```python
from build123d import *

# Parameters (mm, degrees)
BOSS_EXTRUDE1_START = 0.1
SKETCH1_R           = 3.884465816
BOSS_EXTRUDE1_DEPTH = 2.9
SKETCH2_R           = 3.884465816
SKETCH2_R_2         = 1.6
BOSS_EXTRUDE2_DEPTH = 1
SKETCH3_R           = 2.45
SKETCH3_R_2         = 1.6
BOSS_EXTRUDE3_DEPTH = 15.8


with BuildPart() as part:
    # Sketch1 → Boss-Extrude1 (new body)
    with BuildSketch(Plane.XY.offset(BOSS_EXTRUDE1_START)):
        with Locations((-0.001459351, 10.192904416)):
            Circle(SKETCH1_R)
        with BuildLine():
            Line((0.96845111, 13.081919272), (0.60411229, 12.721398629))
            ThreePointArc((0.60411229, 12.721398629), (0.587991908, 12.72520519), (0.571847603, 12.728908977))
            Line((0.571847603, 12.728908977), (0.404173908, 13.213267772))
            Line((0.404173908, 13.213267772), (0.114648145, 12.790310631))
            ThreePointArc((0.114648145, 12.790310631), (0.098098683, 12.790997601), (0.08154518, 12.791579126))
            Line((0.08154518, 12.791579126), (-0.174763937, 13.23545247))
            Line((-0.174763937, 13.23545247), (-0.379012427, 12.765345605))
            ThreePointArc((-0.379012427, 12.765345605), (-0.395392828, 12.762888154), (-0.411757242, 12.760326399))
            Line((-0.411757242, 12.760326399), (-0.747438103, 13.147671554))
            Line((-0.747438103, 13.147671554), (-0.859027247, 12.647405852))
            ThreePointArc((-0.859027247, 12.647405852), (-0.874646558, 12.641892799), (-0.89023043, 12.636280352))
            Line((-0.89023043, 12.636280352), (-1.293150653, 12.953097656))
            Line((-1.293150653, 12.953097656), (-1.308047329, 12.440754022))
            ThreePointArc((-1.308047329, 12.440754022), (-1.322341026, 12.432384623), (-1.336581115, 12.423924333))
            Line((-1.336581115, 12.423924333), (-1.792178114, 12.658763182))
            Line((-1.792178114, 12.658763182), (-1.709843917, 12.152859051))
            ThreePointArc((-1.709843917, 12.152859051), (-1.72229539, 12.141935797), (-1.734677021, 12.130933442))
            Line((-1.734677021, 12.130933442), (-2.226484333, 12.275306147))
            Line((-2.226484333, 12.275306147), (-2.049895036, 11.794126212))
            ThreePointArc((-2.049895036, 11.794126212), (-2.060054255, 11.781043899), (-2.070129925, 11.767897132))
            Line((-2.070129925, 11.767897132), (-2.580372352, 11.816585689))
            Line((-2.580372352, 11.816585689), (-2.315910352, 11.377521046))
            ThreePointArc((-2.315910352, 11.377521046), (-2.323410137, 11.362752503), (-2.330815684, 11.347936481))
            Line((-2.330815684, 11.347936481), (-2.841051735, 11.299181158))
            Line((-2.841051735, 11.299181158), (-2.498275379, 10.918100748))
            ThreePointArc((-2.498275379, 10.918100748), (-2.502844667, 10.902179748), (-2.507312436, 10.886229962))
            Line((-2.507312436, 10.886229962), (-2.999100852, 10.741792904))
            Line((-2.999100852, 10.741792904), (-2.590398969, 10.432469965))
            ThreePointArc((-2.590398969, 10.432469965), (-2.591872615, 10.415971935), (-2.593241129, 10.399464852))
            Line((-2.593241129, 10.399464852), (-3.048807394, 10.16456639))
            Line((-3.048807394, 10.16456639), (-2.588951536, 9.938180659))
            ThreePointArc((-2.588951536, 9.938180659), (-2.587276279, 9.921701881), (-2.585496075, 9.905234109))
            Line((-2.585496075, 9.905234109), (-2.988374839, 9.588364086))
            Line((-2.988374839, 9.588364086), (-2.493985393, 9.453097734))
            ThreePointArc((-2.493985393, 9.453097734), (-2.489221781, 9.437233793), (-2.484357202, 9.421400521))
            Line((-2.484357202, 9.421400521), (-2.819987375, 9.034011444))
            Line((-2.819987375, 9.034011444), (-2.308932865, 8.994753349))
            ThreePointArc((-2.308932865, 8.994753349), (-2.301253067, 8.98007761), (-2.293479931, 8.965451093))
            Line((-2.293479931, 8.965451093), (-2.549730965, 8.521544214))
            Line((-2.549730965, 8.521544214), (-2.040482233, 8.579713266))
            ThreePointArc((-2.040482233, 8.579713266), (-2.030163816, 8.566756147), (-2.019763064, 8.553865027))
            Line((-2.019763064, 8.553865027), (-2.187373379, 8.069484296))
            Line((-2.187373379, 8.069484296), (-1.698336, 8.222978114))
            ThreePointArc((-1.698336, 8.222978114), (-1.6857519, 8.21220792), (-1.673099443, 8.201518114))
            Line((-1.673099443, 8.201518114), (-1.746011165, 7.694170314))
            Line((-1.746011165, 7.694170314), (-1.294860225, 7.937441231))
            ThreePointArc((-1.294860225, 7.937441231), (-1.280465263, 7.929247225), (-1.266018393, 7.921145091))
            Line((-1.266018393, 7.921145091), (-1.241596303, 7.409167093))
            Line((-1.241596303, 7.409167093), (-0.844637572, 7.733422664))
            ThreePointArc((-0.844637572, 7.733422664), (-0.82895202, 7.728100999), (-0.813232885, 7.722879369))
            Line((-0.813232885, 7.722879369), (-0.69235966, 7.224775391))
            Line((-0.69235966, 7.224775391), (-0.363940261, 7.618296176))
            ThreePointArc((-0.363940261, 7.618296176), (-0.347531036, 7.616039191), (-0.331107766, 7.613886788))
            Line((-0.331107766, 7.613886788), (-0.11815208, 7.147659606))
            Line((-0.11815208, 7.147659606), (0.129858055, 7.596222737))
            ThreePointArc((0.129858055, 7.596222737), (0.14639788, 7.597112005), (0.162931705, 7.598106624))
            Line((0.162931705, 7.598106624), (0.460273079, 7.180606903))
            Line((0.460273079, 7.180606903), (0.618910217, 7.66800014))
            ThreePointArc((0.618910217, 7.66800014), (0.634982852, 7.67200352), (0.651029656, 7.676109212))
            Line((0.651029656, 7.676109212), (1.022010025, 7.32242648))
            Line((1.022010025, 7.32242648), (1.085540607, 7.831034163))
            ThreePointArc((1.085540607, 7.831034163), (1.100565143, 7.838006962), (1.115544953, 7.845075337))
            Line((1.115544953, 7.845075337), (1.546756122, 7.567992608))
            Line((1.546756122, 7.567992608), (1.512883986, 8.079432329))
            ThreePointArc((1.512883986, 8.079432329), (1.526317398, 8.089122534), (1.539688805, 8.098898121))
            Line((1.539688805, 8.098898121), (2.015545677, 7.908429889))
            Line((2.015545677, 7.908429889), (1.885495051, 8.404216884))
            ThreePointArc((1.885495051, 8.404216884), (1.896851821, 8.416274264), (1.908131547, 8.428403749))
            Line((1.908131547, 8.428403749), (2.411435415, 8.331434031))
            Line((2.411435415, 8.331434031), (2.189906668, 8.793649267))
            ThreePointArc((2.189906668, 8.793649267), (2.198776332, 8.807638037), (2.207556699, 8.821683028))
            Line((2.207556699, 8.821683028), (2.72011685, 8.821716563))
            Line((2.72011685, 8.821716563), (2.415116608, 9.233654376))
            ThreePointArc((2.415116608, 9.233654376), (2.421178593, 9.249068946), (2.427142255, 9.264521821))
            Line((2.427142255, 9.264521821), (2.93043343, 9.361557396))
            Line((2.93043343, 9.361557396), (2.552985195, 9.708329281))
            ThreePointArc((2.552985195, 9.708329281), (2.556020406, 9.724612528), (2.558951821, 9.74091478))
            Line((2.558951821, 9.74091478), (3.034783766, 9.931445277))
            Line((3.034783766, 9.931445277), (2.598529502, 10.200517994))
            ThreePointArc((2.598529502, 10.200517994), (2.598428238, 10.217081399), (2.598221457, 10.233643822))
            Line((2.598221457, 10.233643822), (3.029396365, 10.510782972))
            Line((3.029396365, 10.510782972), (2.550103437, 10.692431532))
            ThreePointArc((2.550103437, 10.692431532), (2.546869358, 10.70867645), (2.543531855, 10.724900436))
            Line((2.543531855, 10.724900436), (2.914465941, 11.078631708))
            Line((2.914465941, 11.078631708), (2.409457245, 11.166290859))
            ThreePointArc((2.409457245, 11.166290859), (2.403207239, 11.181630157), (2.396859639, 11.196929327))
            Line((2.396859639, 11.196929327), (2.69414638, 11.614467952))
            Line((2.69414638, 11.614467952), (2.181674246, 11.604969464))
            ThreePointArc((2.181674246, 11.604969464), (2.172634204, 11.618848739), (2.163505927, 11.632670142))
            Line((2.163505927, 11.632670142), (2.376400605, 12.098925186))
            Line((2.376400605, 12.098925186), (1.87498711, 11.992612359))
            ThreePointArc((1.87498711, 11.992612359), (1.863483764, 12.004529978), (1.851904729, 12.016374073))
            Line((1.851904729, 12.016374073), (1.972712775, 12.514493863))
            Line((1.972712775, 12.514493863), (1.50048031, 12.315209119))
            ThreePointArc((1.50048031, 12.315209119), (1.48692942, 12.324734349), (1.473318124, 12.334173059))
            Line((1.473318124, 12.334173059), (1.497673221, 12.846154249))
            Line((1.497673221, 12.846154249), (1.071689498, 12.561100258))
            ThreePointArc((1.071689498, 12.561100258), (1.056580829, 12.567888832), (1.041429218, 12.574581017))
            Line((1.041429218, 12.574581017), (0.96845111, 13.081919272))
        make_face(mode=Mode.SUBTRACT)
    extrude(amount=BOSS_EXTRUDE1_DEPTH)

    # Sketch2 → Boss-Extrude2 (add)
    with BuildSketch(Plane.XY.offset(3)):
        with Locations((-0.001459351, 10.192904416)):
            Circle(SKETCH2_R)
        with Locations((-0.001459351, 10.192904416)):
            Circle(SKETCH2_R_2, mode=Mode.SUBTRACT)
    extrude(amount=BOSS_EXTRUDE2_DEPTH)

    # Sketch3 → Boss-Extrude3 (add)
    with BuildSketch(Plane.XY.offset(4)):
        with Locations((-0.001459351, 10.192904416)):
            Circle(SKETCH3_R)
        with Locations((-0.001459351, 10.192904416)):
            Circle(SKETCH3_R_2, mode=Mode.SUBTRACT)
    extrude(amount=BOSS_EXTRUDE3_DEPTH)


solid = part.part
```
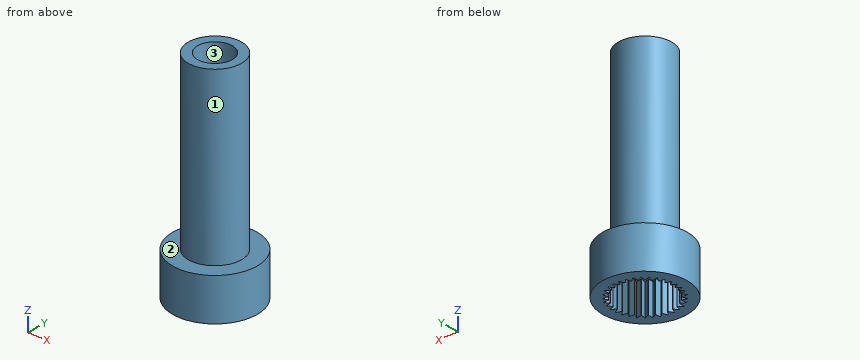
The listing builds one solid part. Answer for the finished solid, in the listing's coordinates (mm). Face numbers are marked on the shaded views. Give positions to 0.01 mm unless a question says otherwise; leave off trailing zeros. Order: outer loops, then holes, each group sorted by start corner. A loop starts at its lowest first (then second) coordinate and runs counter-clockwise, first axis right, second up. Notation, with made-up numbers: (80.25, -23) -> (117.25, -23) arc R25 cw to (117.25, 15) -> close; hole circle Ø3 at (50.25, -18.5). An arc over 180 degrees is marked (long way). Answer as a JSON object with one key per item and string values. Group by question number.
Item 1: The part is cut by section A-A on z = 5.25. Write down the section's boundary in (x, y).
Item 2: Consider L1, parallel to Y at x = 0, z = 13.5; L2, parallel to Z at x = 0, y = 8.5; L3, parallel to Y at x = -0.75, z = 6.5. Determine where each line is inside the solid, lowest interval first. Write a range as from..to.
Item 3: Flat-ended cylindrical pins translate along their axes: pin 1 (1.5 mm diameter, centred on y = 11, z = 17.5, fed in from +X); pin 2 (2.5 mm diameter, centred on x = 0, y = 10.19, fed in from -Z); pin 3 (1.5 mm diameter, centred on y = 11, z = 8.5, fed in from -X). Find the tip coordinate at first contact, or state that the pin passes through.
Item 4: The part is cut by section B-B on x = -3.5. Write down the section's boundary in (y, z), and give its area (3 significant figures).
Item 5: Determine the mould class of the marked faces 1, 2 and 3 for opening direction X: pulls with the +X half, pulls with the -X half, needs draft (parallel to the pull), parting line crosses it, or undercut.
Result set:
{
 "1": {"outline": "circle Ø4.9 at (0, 10.19); hole circle Ø3.2 at (0, 10.19)"},
 "2": {"L1": "7.74..8.59, 11.79..12.64", "L2": "3..19.8", "L3": "7.86..8.78, 11.61..12.53"},
 "3": {"pin 1": "x = 2.45", "pin 2": "through", "pin 3": "x = -2.45"},
 "4": {"outline": "(8.5, 0.1) -> (11.88, 0.1) -> (11.88, 4) -> (8.5, 4) -> close", "area": "13.2 mm²"},
 "5": {"face 1": "parting line crosses it", "face 2": "needs draft", "face 3": "undercut"}
}
